Geometry check sheet. Reference: the model listing, model coordinates, mm. A direction names the side the tool comes from. Give positions to 0.01 mm unless a question says otherwise; leave off trailing zeros. Loops run counter-clockwise (first coordinate to the right, second up) from the corner with the lowest first, then second, coordinate; pieces in that order, holes last. Notation, with made-up numbers: (-29.75, -17) -> (0.25, -17) arc R20 ccw to (0.25, -9) -> close; hole circle Ø9 at (18.5, 85.5). An arc over 180 degrees is marked (long way). Write item = value, one per line.
```python
from build123d import *

# Parameters (mm, degrees)
F0_R          = 8.2355585824
F1_ANGLE_BACK = 15
F1_ANGLE      = 30
F2_W          = 15
F2_H          = 15
F3_DEPTH      = 25
F4_W          = 15.1891945861
F4_H          = 12.1442461386
F5_DEPTH      = 80


with BuildPart() as f1:
    # F0 (on Right) → F1 (revolve)
    with BuildSketch(Plane.YZ, mode=Mode.PRIVATE) as f1_sk:
        Circle(F0_R)
    revolve(f1_sk.sketch.rotate(Axis((0, -74.6255367994, -4.2161336169), (0, 0, -1)), -F1_ANGLE_BACK), axis=Axis((0, -74.6255367994, -4.2161336169), (0, 0, -1)), revolution_arc=F1_ANGLE)

    # F2 (on Front) → F3 (join)
    with BuildSketch(Plane.XZ):
        with Locations((0, -0.4352101311)):
            Rectangle(F2_W, F2_H)
    extrude(amount=-F3_DEPTH)

    # F4 (on Top) → F5 (join)
    with BuildSketch(Plane.XY):
        with Locations((-0.0722266268, 19.7329348885)):
            Rectangle(F4_W, F4_H)
    extrude(amount=F5_DEPTH)


solid = f1.part
```
Item 1: Section check B-B, the plane z = 37.5. Record the cut outline in (x, y).
Answer:
outline = (-7.67, 13.66) -> (7.52, 13.66) -> (7.52, 25.81) -> (-7.67, 25.81) -> close
Item 2: Tool access check on faces 3 (the flat face through (0, 20, 80)), 4 (the flat face through (0, 25, -4)). Record the directions out of +Z, -Z, +X, -X, +Y, -Y that give a thin tool (end or side, any length) a straight path to the whole face; none if there is none.
Answer:
face_3 = +Z, +X, -X, +Y, -Y
face_4 = -Z, +X, -X, +Y
Item 3: Draft check along Y on faces 1 (the flat face through (-7.5, 13, -2)), 2 (the flat face through (-19.285, -2.654, 0.115)). Enter one of: +Y half, -Y half, draft (parallel to the pull), parting line (faces both ways), or undercut.
Answer:
face_1 = undercut
face_2 = -Y half
Item 4: Gauge pin test, flat ends, axial feed: pin 1 (10 mm diameter, centred on x = 8.5, z = 9.5, fed in from +Y); pin 2 (9.5 mm diameter, centred on y = 21, z = 39.5, fed in from -X); pin 3 (3 mm diameter, centred on y = 12.5, z = 42, fed in from +X); pin 4 (6 mm diameter, centred on x = 13.5, y = 3.5, fed in from +Z). Record the tip position at first contact, or that the pin passes through.
Answer:
pin_1 = 25.81
pin_2 = -7.67
pin_3 = 7.52
pin_4 = 8.07
Item 5: Thickness scan on L1, parallel to Y at x = -4, z = 36; L2, parallel to Y at x = 4, z = 1.5; L3, parallel to Z at x = -5, y = 7.5. Record the ranges inside material, lowest first. Write a range as [from, to].
Answer:
L1 = [13.66, 25.81]
L2 = [-8.22, 25.81]
L3 = [-7.94, 7.06]
